```python
from build123d import *

# Parameters (mm, degrees)
ESQUISSE2_R                  = 2.25
ENL_V_MAT_EXTRU_1_DEPTH      = 47.491934784
R_P_TITION_CIRCULAIRE1_COUNT = 3


with BuildPart() as part:
    # Esquisse1 → Révolution1 (revolve)
    with BuildSketch(Plane.XY):
        Polygon((-10, -7), (-10, -5.5), (-20, -5.5), (-20, 3.5), (-23, 3.5), (-23.5, 3), (-23.5, 0), (-32.5, 0), (-32.5, -5), (-22, -5), (-22, -7), align=None)
    revolve(axis=Axis((0, 39.107095159, 0), (0, -1, 0)))

    # Esquisse2 → Enlèv. mat.-Extru.1 (cut, through all)
    with BuildSketch(Plane(origin=(0, 0, 0), x_dir=(-1, 0, 0), z_dir=(0, 1, 0))):
        with Locations((0, 28)):
            Circle(ESQUISSE2_R)
    enl_v_mat_extru_1 = extrude(amount=-ENL_V_MAT_EXTRU_1_DEPTH, mode=Mode.SUBTRACT)

    # Répétition circulaire1: Enlèv. mat.-Extru.1 ×3 about axis
    r_p_tition_circulaire1_axis = Axis((0, 0, 0), (0, 1, 0))
    for i in range(1, R_P_TITION_CIRCULAIRE1_COUNT):
        add(enl_v_mat_extru_1.rotate(r_p_tition_circulaire1_axis, i * 360 / R_P_TITION_CIRCULAIRE1_COUNT), mode=Mode.SUBTRACT)


solid = part.part
```
Check sheet for the modelled part. Datum: model origin and axes. Units: mm. A direction names the side the tool comes from. Give positions to 0.01 mm unless a question says otherwise; leave off trailing zeros. Write each loop counter-clockwise with the first axis right and the second up, starting at its lowest first coordinate (ties: lowest second). Pieces come first, ordered by that corner, then holes.
Item 1: Cross-section at B-B (y = -4). Enter the section's corners in (x, z), and give its area (3 significant figures).
Item 2: Access from +Z, -Z, +X, -X, +Y, -Y to the whole of each face (thin tool, end or side, straight path). Record for faces 5 (the face through (-21.2, -5, 6.8)), 6 (the face through (-22.4, 1.5, -7.1)), 7 (the face through (-25.287, -2.465, -15.996)).
Item 3: Draft check along X on faces 1 (the face through (2.17, -6.24, 9.76)), 2 (the face through (4.769, -6.014, 21.477)), 3 (the face through (0, 0, -24)), 4 (the face through (0.488, -2.465, 25.804)). Enter one of: released by +X, released by -X, zero draft, split by the parting line, or undercut.
Item 4: Cross-section at D-D (z = -25.5). Enter the section's corners in (x, y), and give its area (3 significant figures).
Item 5: Gauge pin test, flat ends, axial feed: pin 1 (4 mm diameter, centred on y = -3.5, z = -18, fed in from +X); pin 2 (1.5 mm diameter, centred on x = 24, y = -4.5, fed in from +Z); pin 3 (6 mm diameter, centred on x = -4, y = 1, fed in from +Z); pin 4 (3.5 mm diameter, centred on x = 24.25, z = -14, fed in from +Y). Record the tip position at first contact, or that the pin passes through.
Item 6: Cross-section at A-A (x = 0). Enter the section's corners in (y, z).
Item 7: Cross-section at C-C (z = -14). Count the separate pieces of the cut face and the enclosed holes in it, and give its area (3 significant figures).
Item 8: Scan lines: L1, parallel to Z at x = 0, y = -2.5; L2, parallel to X at y = -2.5, z = 0; L3, parallel to X at y = -5.8, z = 0. Record each from-to range of solid material in increasing order.
Report:
1. outline: circle Ø65 at (0, 0); hole circle Ø4.5 at (-24.25, -14); hole circle Ø40 at (0, 0); hole circle Ø4.5 at (0, 28); hole circle Ø4.5 at (24.25, -14)
1. area: 2,010 mm2
2. face 5: -Y
2. face 6: +Y
2. face 7: +Y, -Y
3. face 1: undercut
3. face 2: split by the parting line
3. face 3: zero draft
3. face 4: undercut
4. outline: (-20.15, -5) - (20.15, -5) - (20.15, 0) - (-20.15, 0) - close
4. area: 201 mm2
5. pin 1: stops at x = 28.29
5. pin 2: stops at z = 22.71
5. pin 3: stops at z = 32.48
5. pin 4: passes through
6. outline: (-7, -22) - (-5, -22) - (-5, -32.5) - (0, -32.5) - (0, -23.5) - (3, -23.5) - (3.5, -23) - (3.5, -20) - (-5.5, -20) - (-5.5, -10) - (-7, -10) - close; (-7, 10) - (-5.5, 10) - (-5.5, 20) - (3.5, 20) - (3.5, 23) - (3, 23.5) - (0, 23.5) - (0, 25.75) - (-5, 25.75) - (-5, 22) - (-7, 22) - close; (-5, 30.25) - (0, 30.25) - (0, 32.5) - (-5, 32.5) - close
7. separate pieces: 3
7. enclosed holes: 0
7. area: 191 mm2
8. L1: z = -32.5 to -20, 20 to 25.75, 30.25 to 32.5
8. L2: x = -32.5 to -20, 20 to 32.5
8. L3: x = -22 to -10, 10 to 22
